```python
from build123d import *

# Parameters (mm, degrees)
SKETCH1_R      = 3.9624
EXTRUDE1_DEPTH = 2.2098
FILLET1_R      = 1.524
SKETCH2_R      = 2.0828
EXTRUDE2_DEPTH = 19.05
EXTRUDE3_DEPTH = 1.016


with BuildPart() as part:
    # Sketch1 → Extrude1 (new body)
    with BuildSketch(Plane.XY):
        Circle(SKETCH1_R)
    extrude(amount=EXTRUDE1_DEPTH)

    # Fillet1
    fillet1_edges = [part.edges().sort_by_distance(p)[0] for p in [
        (-3.9624, 0, 0),
    ]]
    fillet(fillet1_edges, radius=FILLET1_R)

    # Sketch2 → Extrude2 (add)
    with BuildSketch(Plane.XY.offset(2.2098)):
        Circle(SKETCH2_R)
    extrude(amount=EXTRUDE2_DEPTH)

    # Sketch3 → Extrude3 (cut)
    with BuildSketch(Plane(origin=(0, 0, 0), x_dir=(-1, 0, 0), z_dir=(0, 0, -1))):
        Polygon((0.709024608, 1.177879999), (-0.665561698, 1.202973322), (-1.374586306, 0.025093323), (-0.709024608, -1.177879999), (0.665561698, -1.202973322), (1.374586306, -0.025093323), align=None)
    extrude(amount=-EXTRUDE3_DEPTH, mode=Mode.SUBTRACT)


solid = part.part
```
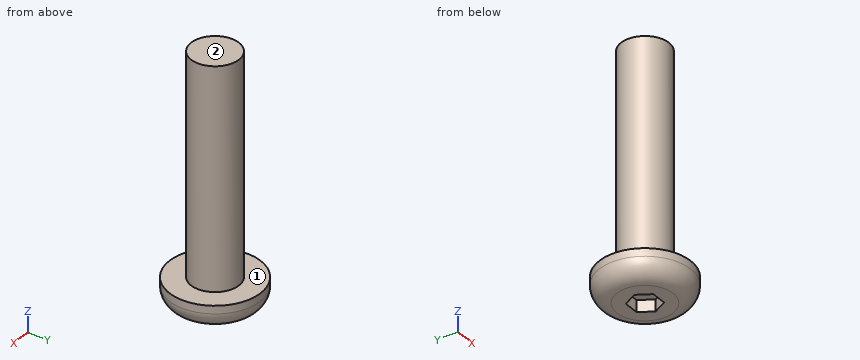
The model under review builds one solid part; all positions refer to its coordinate system, in mm. Face numbers are marked on the shaded views. A direction names the side the tool comes from. Round coordinates to 2 decimals unless told otherwise and drop trailing zeros. Write each loop counter-clockwise with the first axis right and the second up, starting at its lowest first coordinate (ties: lowest second). Pieces come first, ordered by that corner, then holes. Notation, with made-up numbers: (-17.75, 76.5) - (-6.75, 76.5) arc R25 cw to (-6.75, 106.5) - close; hole circle Ø5 at (-5, 32). An arc over 180 degrees is marked (long way). One line per question, with ' | ' between items.
Item 1: Add section B-B, the plane x = 0. Give the boundary of the cut face in (y, z), then the cut area to 3 significant figures.
Resolved:
outline: (-3.96, 1.52) arc R1.52 ccw to (-2.44, 0) - (-1.19, 0) - (-1.19, 1.02) - (1.19, 1.02) - (1.19, 0) - (2.44, 0) arc R1.52 ccw to (3.96, 1.52) - (3.96, 2.21) - (2.08, 2.21) - (2.08, 21.26) - (-2.08, 21.26) - (-2.08, 2.21) - (-3.96, 2.21) - close | area: 93.5 mm2
Item 2: To check wall thickness, follow probe 1 along Z at (x, y) = (-1.5, 2); probe 2 along Z at (x, y) = (0, 0.5); probe 3 along Y at (x, z) = (0, 14.75). State the ranges of each line that lie inside material, in increasing order.
Resolved:
probe 1: z = 0 to 2.21 | probe 2: z = 1.02 to 21.26 | probe 3: y = -2.08 to 2.08
Item 3: For the marked faces 1 and 2, list the 3-axis set-ups (+Z, -Z, +X, -X, +Y, -Y) from which the entire face can be reached by the end or side of a thin tool; tool diameter is ignored.
Resolved:
face 1: +Z | face 2: +Z, +X, -X, +Y, -Y
Item 4: Add section A-A, the plane z = 10.25. Give the boundary of the cut face in (x, y).
Resolved:
outline: circle Ø4.17 at (0, 0)
Item 5: For P1, Ø1, axis at x = -2.5, y = -0.5, coming from the +Z side; P2, Ø1.5, axis at y = -2, z = 5, coming from the +X side; P3, Ø3, axis at x = -3, z = 14, coming from the +Y side (3 decimals); P4, Ø0.7, axis at x = -0.5, y = -0.5, coming from the -Z side, all flat-tipped, find the tip position at first contact; note any pin that passes through.
Resolved:
P1: stops at z = 21.26 | P2: stops at x = 1.67 | P3: stops at y = 1.445 | P4: stops at z = 1.02
